Check sheet for the modelled part. Datum: model origin and axes. Units: mm. Give positions to 0.01 mm unless a question says otherwise; leave off trailing zeros. Loops run counter-clockwise (first coordinate to the right, second up) from the corner with the lowest first, then second, coordinate; pieces in that order, holes last. Notation, with made-up numbers: M 67.5,33 L 102.5,33 A8 ccw 102.5,38 Z; hole C 35.25,-10.5 d1. An arc over 180 degrees is marked long. Put each result on its own line as item: value. Start each with the question number.
```python
from build123d import *
from build123d.topology import SkipClean

# Parameters (mm, degrees)
SKETCH2_W           = 25.4
SKETCH2_H           = 25.4
BOSS_EXTRUDE1_DEPTH = 736.6
SKETCH4_R           = 3.175
SKETCH4_R_2         = 1.984375
CUT_EXTRUDE1_DEPTH  = 736.6
SKETCH5_R           = 1.984375
CUT_EXTRUDE2_DEPTH  = 736.6
CUT_EXTRUDE3_DEPTH  = 736.6


with BuildPart() as part:
    # Sketch2 → Boss-Extrude1 (new body)
    with BuildSketch(Plane.XY):
        with Locations((12.7, 12.7)):
            Rectangle(SKETCH2_W, SKETCH2_H)
    extrude(amount=BOSS_EXTRUDE1_DEPTH)

    # Sketch4 → Cut-Extrude1 (cut)
    with BuildSketch(Plane(origin=(0, 25.4, 0), x_dir=(1, 0, 0), z_dir=(0, 1, 0))):
        with Locations(Location((12.7, -9.525, 0), (0, 0, 270))):
            Circle(SKETCH4_R)
        with Locations(Location((12.7, -53.975, 0), (0, 0, 270))):
            Circle(SKETCH4_R)
        with Locations(Location((12.7, -723.9, 0), (0, 0, 270))):
            Circle(SKETCH4_R_2)
    extrude(amount=-CUT_EXTRUDE1_DEPTH, mode=Mode.SUBTRACT)

    # Sketch5 → Cut-Extrude2 (cut)
    with BuildSketch(Plane(origin=(25.4, 0, 0), x_dir=(0, 0, -1), z_dir=(1, 0, 0))):
        with Locations((-723.9, 12.7)):
            Circle(SKETCH5_R)
    extrude(amount=-CUT_EXTRUDE2_DEPTH, mode=Mode.SUBTRACT)

    # Sketch6 → Cut-Extrude3 (cut)
    with SkipClean():  # the faces are left unmerged after this step: merging them gives an invalid solid
        with BuildSketch(Plane.XY.offset(736.6)):
            with BuildLine():
                Line((0, 25.4), (0, 12.7))
                ThreePointArc((0, 12.7), (3.719743879, 21.680256121), (12.7, 25.4))
                Line((12.7, 25.4), (0, 25.4))
            make_face()
            with BuildLine():
                ThreePointArc((12.7, 25.4), (21.680256121, 21.680256121), (25.4, 12.7))
                Line((25.4, 12.7), (25.4, 25.4))
                Line((25.4, 25.4), (12.7, 25.4))
            make_face()
            with BuildLine():
                Line((25.4, 0), (25.4, 12.7))
                ThreePointArc((25.4, 12.7), (21.680256121, 3.719743879), (12.7, 0))
                Line((12.7, 0), (25.4, 0))
            make_face()
            with BuildLine():
                ThreePointArc((12.7, 0), (3.719743879, 3.719743879), (0, 12.7))
                Line((0, 12.7), (0, 0))
                Line((0, 0), (12.7, 0))
            make_face()
        extrude(amount=-CUT_EXTRUDE3_DEPTH, mode=Mode.SUBTRACT)


solid = part.part
```
Q1. Thickness scan on line 1 along Z through (x, y) = (12.7, 10); line 2 along Z through (x, y) = (12, 23); line 3 along Z through (x, y) = (3.75, 12.7). Record the ranges inside material, lowest first. Write a range as [from, to].
Q2. Section check B-B, the plane y = 20.5. Record the cut outline in (x, z) (3 decimals).
Q3. Section check A-A, the plane x = 5. Record the cut outline in (y, z), then the cut area to 3 significant figures.
Q4. Depth check by flat-ended pin: P1, Ø1, axis at y = 3, z = 398.5, coming from the +X side (3 decimals); P2, Ø3, axis at x = 12.7, z = 723.9, coming from the +Y side; P3, Ø8, axis at y = 21.5, z = 146, coming from the +X side; P4, Ø2, axis at x = 8, z = 198.5, coming from the +Y side. Enter the tip coordinate at first touch or a pass-through.
Q5. Section check C-C, the plane z = 429. Record the cut outline in (x, y), then the cut area to 3 significant figures.
Found:
1. line 1: z = [0, 6.35], [12.7, 50.8], [57.15, 721.92], [725.88, 736.6]
1. line 2: z = [0, 6.43], [12.62, 50.88], [57.07, 722.04], [725.76, 736.6]
1. line 3: z = [0, 721.92], [725.88, 736.6]
2. outline: M 2.678,0 L 22.722,0 L 22.722,736.6 L 2.678,736.6 Z; hole C 12.7,9.525 d6.35; hole C 12.7,53.975 d6.35; hole C 12.7,723.9 d3.969
3. outline: M 2.6,0 L 22.8,0 L 22.8,736.6 L 2.6,736.6 Z; hole C 12.7,723.9 d3.97
3. area: 14,900 mm^2
4. P1: stops at x = 21.455
4. P2: passes through
4. P3: stops at x = 24.46
4. P4: stops at y = 24.85
5. outline: C 12.7,12.7 d25.4
5. area: 507 mm^2
